Input: part model. Units: mm. Frame: model coordinates. A direction names the side the tool comes from. Give positions to 0.01 mm unless a question says otherwise; leave off trailing zeros. Loops run counter-clockwise (first coordinate to the right, second up) from the corner with the lowest first, then second, coordinate; pieces in that order, holes last. Notation, with made-up numbers: M 66.25,70.5 L 87.25,70.5 A30 ccw 87.25,106.5 Z; hole C 7,-25 d5. An arc over 180 degrees is marked long. Answer as a JSON object with one key per item and string values. Group by question number.
```python
from build123d import *

# Parameters (mm, degrees)
SKETCH3_R   = 29.972
SKETCH3_R_2 = 19.05


with BuildPart() as part:
    # Sketch1 → Revolve1 (revolve)
    with BuildSketch(Plane.XY, mode=Mode.PRIVATE) as revolve1_sk:
        Polygon((-62.23, -29.972), (-26.67, -29.972), (-26.67, -24.0538), (-62.23, -24.2824), align=None)
    revolve(revolve1_sk.sketch.rotate(Axis((-62.23, 0, 0), (1, 0, 0)), 270), axis=Axis((-62.23, 0, 0), (1, 0, 0)))


with BuildPart() as body_2:
    # Sketch2 → Revolve2 (revolve)
    with BuildSketch(Plane.XY, mode=Mode.PRIVATE) as revolve2_sk:
        Polygon((24.2824, 62.23), (24.0538, 26.67), (29.972, 26.67), (29.972, 62.23), align=None)
    revolve(revolve2_sk.sketch.rotate(Axis((0, 0, 0), (0, 1, 0)), 90), axis=Axis((0, 0, 0), (0, 1, 0)))


with BuildPart() as sweep1_tool:
    # Sweep1: sweep along a path in Sketch4
    with BuildLine(Plane.XY) as sweep1_path:
        ThreePointArc((-26.67, 0), (-7.811462, 7.811462), (0, 26.67))
    # Sketch3 → Sweep1 (sweep)
    with BuildSketch(Plane(origin=(-26.67, 0, 0), x_dir=(0, 0, -1), z_dir=(1, 0, 0))):
        Circle(SKETCH3_R)
        Circle(SKETCH3_R_2, mode=Mode.SUBTRACT)
    sweep(path=sweep1_path.line)


with BuildPart() as part_1:
    add(part.part)


with BuildPart() as part_2:
    # Sweep1: joined with sweep1_tool
    add(part_1.part.fuse(sweep1_tool.part, body_2.part, tol=0.00001))


solid = part_2.part
```
1. Reachability of faces 1 (the flat face through (-7, 26.67, -18)), 2 (the cylindrical face through (-44.201, -29.717, -3.902)) from +Z, -Z, +X, -X, +Y, -Y: full face, straight path, thin tool, end or side. Return the list, or none.
2. Mould query, pull axis X, two halves, no side actions, for faces 3 (the flat face through (-25, 62.23, 0)), 4 (the flat face through (-62.23, -25, 0)), 5 (the conical face through (-7.26, 44.2, -23.05)). Classes: pulls with the +X half, pulls with the -X half, needs draft (parallel to the pull), parting line crosses it, or undercut.
3. Material intervals for L1, parallel to Y at x = -26.5, z = 0; L2, parallel to Z at x = -6, y = 58.5; L3, parallel to Z at x = 13, y = 51, sorted ascending.
4. Section B-B (x = -37). Output: boundary loops of the cut face in (y, z), then the cut area to 3 significant figures.
5. Section A-A (y = 54). Output: boundary loops of the cut face in (x, z).
6. First-contact query: P1, Ø4, axis at x = 20.5, y = -2.5, coming from the +Z side; P2, Ø3, axis at x = -13.5, z = 8.5, coming from the -Y side; P3, Ø3, axis at x = -8, y = -9, coming from the +Z side. Flat tips, straight axial feed; report the tip coordinate or a pass-through.
Geometry results:
{
 "1": {"face 1": "+Y", "face 2": "-X"},
 "2": {"face 3": "needs draft", "face 4": "pulls with the -X half", "face 5": "undercut"},
 "3": {"L1": "-29.97 to -19.05, 19.05 to 62.23", "L2": "-29.37 to -23.5, 23.5 to 29.37", "L3": "-27.01 to -20.42, 20.42 to 27.01"},
 "4": {"outline": "C 0,0 d59.94; hole C 0,0 d48.24", "area": "994 mm2"},
 "5": {"outline": "C 0,0 d59.94; hole C 0,0 d48.46"},
 "6": {"P1": "z = 13.44", "P2": "y = -27.7", "P3": "z = 27.43"}
}
